The listing builds one solid part. Answer for the finished solid, in the listing's coordinates (mm). Face numbers are marked on the shaded views. A direction names the side the tool comes from. Give positions to 0.01 mm unless a question says otherwise; leave off trailing zeros. Order: outer loops, then holes, each group sorted by start corner. A loop starts at its lowest first (then second) coordinate and runs counter-clockwise, first axis right, second up. Notation, with made-up numbers: (1, 24) - (38, 24) arc R11 cw to (38, 34) - close; hole circle Ø7 at (33, -32). An arc over 180 degrees is marked (long way). Answer in a Markdown table with one row per item.
from build123d import *

# Parameters (mm, degrees)
SKETCH_4_R      = 19.479021456
SKETCH_4_R_2    = 1
EXTRUDE_1_DEPTH = 1.2
EXTRUDE_2_DEPTH = 11


with BuildPart() as part:
    # 草图4 → 凸台-拉伸1 (new body)
    with BuildSketch(Plane.XY):
        with Locations((-13.402062784, 0.00779119)):
            Circle(SKETCH_4_R)
        with Locations((-25.902062784, 12.50779119)):
            Circle(SKETCH_4_R_2, mode=Mode.SUBTRACT)
        with Locations((-0.902062784, 12.50779119)):
            Circle(SKETCH_4_R_2, mode=Mode.SUBTRACT)
        with Locations((-0.902062784, -12.49220881)):
            Circle(SKETCH_4_R_2, mode=Mode.SUBTRACT)
        with Locations((-25.902062784, -12.49220881)):
            Circle(SKETCH_4_R_2, mode=Mode.SUBTRACT)
        with BuildLine():
            Line((-0.421681224, -10.144442196), (-9.866508066, -0.699336529))
            ThreePointArc((-9.866508066, -0.699336529), (-10.159390847, 0.007774575), (-9.866487191, 0.714877033))
            Line((-9.866487191, 0.714877033), (-0.421408953, 10.159676447))
            ThreePointArc((-0.421408953, 10.159676447), (3.076958671, 0.007570212), (-0.421681224, -10.144442196))
        make_face(mode=Mode.SUBTRACT)
        with BuildLine():
            Line((-3.249794328, 12.988145321), (-12.707997878, 3.55452659))
            ThreePointArc((-12.707997878, 3.55452659), (-13.414834543, 3.262553175), (-14.121290651, 3.555446182))
            Line((-14.121290651, 3.555446182), (-23.554139641, 12.988295172))
            ThreePointArc((-23.554139641, 12.988295172), (-13.401941164, 16.486812646), (-3.249794328, 12.988145321))
        make_face(mode=Mode.SUBTRACT)
        with BuildLine():
            Line((-26.382444344, 10.160024576), (-16.937617502, 0.714918908))
            ThreePointArc((-16.937617502, 0.714918908), (-16.64473472, 0.007807804), (-16.937638376, -0.699294654))
            Line((-16.937638376, -0.699294654), (-26.382716615, -10.144094068))
            ThreePointArc((-26.382716615, -10.144094068), (-29.881084239, 0.008012168), (-26.382444344, 10.160024576))
        make_face(mode=Mode.SUBTRACT)
        with BuildLine():
            Line((-23.554331239, -12.972562941), (-14.108248776, -3.55103379))
            ThreePointArc((-14.108248776, -3.55103379), (-13.402062784, -3.259060163), (-12.695876792, -3.55103379))
            Line((-12.695876792, -3.55103379), (-3.249794328, -12.972562941))
            ThreePointArc((-3.249794328, -12.972562941), (-13.402062784, -16.471230267), (-23.554331239, -12.972562941))
        make_face(mode=Mode.SUBTRACT)
    extrude(amount=EXTRUDE_1_DEPTH)

    # 草图5 → 凸台-拉伸2 (add)
    with BuildSketch(Plane.XY.offset(1.2)):
        with BuildLine():
            Line((-17.902062784, -15.844910415), (-18.311674484, -17.287899762))
            ThreePointArc((-18.311674484, -17.287899762), (-13.402062784, -17.971230267), (-8.492451083, -17.287899762))
            Line((-8.492451083, -17.287899762), (-8.902062784, -15.844910415))
            ThreePointArc((-8.902062784, -15.844910415), (-13.402062784, -16.471230267), (-17.902062784, -15.844910415))
        make_face()
        with BuildLine():
            Line((-29.254764388, -4.49220881), (-30.697753735, -4.901820511))
            ThreePointArc((-30.697753735, -4.901820511), (-31.38108424, 0.00779119), (-30.697753735, 4.91740289))
            Line((-30.697753735, 4.91740289), (-29.254764388, 4.50779119))
            ThreePointArc((-29.254764388, 4.50779119), (-29.88108424, 0.00779119), (-29.254764388, -4.49220881))
        make_face()
        with BuildLine():
            Line((-17.902062784, 15.860492794), (-18.311674484, 17.303482141))
            ThreePointArc((-18.311674484, 17.303482141), (-13.402062784, 17.986812646), (-8.492451083, 17.303482141))
            Line((-8.492451083, 17.303482141), (-8.902062784, 15.860492794))
            ThreePointArc((-8.902062784, 15.860492794), (-13.402062784, 16.486812646), (-17.902062784, 15.860492794))
        make_face()
        with BuildLine():
            Line((2.450638821, 4.50779119), (3.893628168, 4.91740289))
            ThreePointArc((3.893628168, 4.91740289), (4.576958673, 0.00779119), (3.893628168, -4.901820511))
            Line((3.893628168, -4.901820511), (2.450638821, -4.49220881))
            ThreePointArc((2.450638821, -4.49220881), (3.076958673, 0.00779119), (2.450638821, 4.50779119))
        make_face()
    extrude(amount=EXTRUDE_2_DEPTH)


solid = part.part
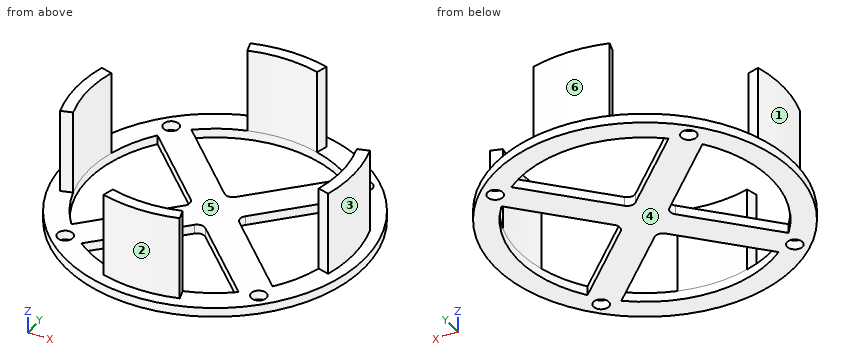
Item 1: Find section B-B on y = 9.5. Write down the section's boundary in (x, z), then the cut area to 3 significant figures.
Answer block:
| item | result |
|---|---|
| outline | (-30.41, 0) - (-26.87, 0) - (-26.87, 1.2) - (-30.41, 1.2) - close; (-25.72, 0) - (-20.07, 0) - (-20.07, 1.2) - (-25.72, 1.2) - close; (-6.75, 0) - (-1.08, 0) - (-1.08, 1.2) - (-6.75, 1.2) - close; (0.07, 0) - (3.61, 0) - (3.61, 1.2) - (0.07, 1.2) - close |
| area | 22.1 mm² |
Item 2: Find section C-C on y = 1.5. Write down the section's boundary in (x, z).
Answer block:
| item | result |
|---|---|
| outline | (-32.82, 0) - (-29.81, 0) - (-29.81, 12.2) - (-31.32, 12.2) - (-31.32, 1.2) - (-32.82, 1.2) - close; (-17.72, 0) - (-9.08, 0) - (-9.08, 1.2) - (-17.72, 1.2) - close; (3.01, 0) - (6.02, 0) - (6.02, 1.2) - (4.51, 1.2) - (4.51, 12.2) - (3.01, 12.2) - close |
Item 3: Consider line 1 (X direction, y = 2, z = 8.5); line 2 (X direction, y = 0, z = 8); line 3 (Z direction, x = -11, y = 5). Determine where each line is inside the solid, lowest interval first.
Answer block:
| item | result |
|---|---|
| line 1 | -31.27 to -29.76, 2.96 to 4.47 |
| line 2 | -31.38 to -29.88, 3.08 to 4.58 |
| line 3 | 0 to 1.2 |
Item 4: Find section A-A on z = 8. Write down the section's boundary in (x, y).
Answer block:
| item | result |
|---|---|
| outline | (-30.7, -4.9) - (-29.25, -4.49) arc R16.48 cw to (-29.25, 4.51) - (-30.7, 4.92) arc R17.98 ccw to start; (-18.31, -17.29) arc R17.98 ccw to (-8.49, -17.29) - (-8.9, -15.84) arc R16.48 cw to (-17.9, -15.84) - close; (-18.31, 17.3) - (-17.9, 15.86) arc R16.48 cw to (-8.9, 15.86) - (-8.49, 17.3) arc R17.98 ccw to start; (2.45, -4.49) - (3.89, -4.9) arc R17.98 ccw to (3.89, 4.92) - (2.45, 4.51) arc R16.48 cw to start |
Item 5: Each of these flat-tipped pins is pushed along its axis until it touches: P1, Ø1.6, axis at x = -25.9, y = 12.51, coming from the -Z side; P2, Ø2.5, axis at x = -25.9, y = -12.49, coming from the +Z side; P3, Ø1.5, axis at x = -9, z = 10, coming from the -Y side; P4, Ø6, axis at x = -28, z = 10, coming from the +Y side. Where does it stop, or does it pass through?
Answer block:
| item | result |
|---|---|
| P1 | through |
| P2 | z = 1.2 |
| P3 | y = -17.6 |
| P4 | y = 4.92 |
Item 6: Which of the six approach directions +Z, -Z, +X, -X, +Y, -Y give full straight-line access (tool end or side, diameter ignored) to the marked faces 1, 2 and 3?
Answer block:
| item | result |
|---|---|
| face 1 | +Z, -X |
| face 2 | +Z, -Y |
| face 3 | +Z, +X |
Item 7: Determine the mould class of the marked faces 4, 5 and 6 for opening direction X: pulls with the +X half, pulls with the -X half, needs draft (parallel to the pull), parting line crosses it, or undercut.
Answer block:
| item | result |
|---|---|
| face 4 | needs draft |
| face 5 | undercut |
| face 6 | parting line crosses it |
